```python
from build123d import *

# Parameters (mm, degrees)
BOSS_EXTRUDE1_DEPTH = 10
SKETCH4_R           = 7.5
CUT_EXTRUDE1_DEPTH  = 11
CHAMFER1_SIZE       = 1


with BuildPart() as part:
    # Sketch3 → Boss-Extrude1 (new body)
    with BuildSketch(Plane(origin=(0, 0, 0), x_dir=(1, 0, 0), z_dir=(0, 1, 0))):
        Polygon((-11, 6.350852961), (-11, -6.350852961), (0, -12.701705922), (11, -6.350852961), (11, 6.350852961), (0, 12.701705922), align=None)
    extrude(amount=BOSS_EXTRUDE1_DEPTH)

    # Sketch4 → Cut-Extrude1 (cut, through all)
    with BuildSketch(Plane(origin=(0, 10, 0), x_dir=(1, 0, 0), z_dir=(0, 1, 0))):
        Circle(SKETCH4_R)
    extrude(amount=-CUT_EXTRUDE1_DEPTH, mode=Mode.SUBTRACT)

    # Chamfer1
    chamfer1_edges = [part.edges().sort_by_distance(p)[0] for p in [
        (-7.5, 0, 0),
        (-7.5, 10, 0),
    ]]
    chamfer(chamfer1_edges, length=CHAMFER1_SIZE)

    # Sketch5 → Cut-Revolve1 (revolve, cut)
    with BuildSketch(Plane(origin=(0, 0, 0), x_dir=(0, 0, -1), z_dir=(1, 0, 0))):
        Polygon((-12.701705922, 10), (-12.701705922, 8.8), (-11.201705922, 10), align=None)
        Polygon((-12.701705922, 0), (-12.701705922, 1.2), (-11.201705922, 0), align=None)
    revolve(axis=Axis((0, 13.174691504, 0), (0, -1, 0)), mode=Mode.SUBTRACT)


solid = part.part
```
Geometry check sheet. Reference: the model listing, model coordinates, mm. Coordinates: 2 decimals unless noted, no trailing zeros. Loops run counter-clockwise (first coordinate to the right, second up) from the corner with the lowest first, then second, coordinate; pieces in that order, holes last. Notation, with made-up numbers: (13, 21.25) - (28, 21.25) arc R27 cw to (28, 37.25) - close; hole circle Ø10 at (-38.75, -18.5). An arc over 180 degrees is marked (long way). One line per item, written item: value. Start each with the question number.
(1) Depth check by flat-ended pin: P1, Ø5, axis at x = -4, z = 3.5, coming from the -Y side; P2, Ø1, axis at x = -5, z = 5.5, coming from the -Y side. Enter the tip coordinate at first touch or a pass-through.
(2) Cross-section at B-B on y = 2.5. Enter the section's corners in (x, z).
(3) Cross-section at A-A on z = 0. Enter the section's corners in (x, y).
(4) Material ranges on line 1 (X direction, y = 3.5, z = 0); line 2 (Z direction, x = 3.5, y = 2.75); line 3 (Z direction, x = -6.25, y = 6.5), recorded low to high. Write a range as [from, to].
Results below:
1. P1: stops at y = 0.68
1. P2: stops at y = 0.57
2. outline: (-11, -6.35) - (0, -12.7) - (11, -6.35) - (11, 6.35) - (0, 12.7) - (-11, 6.35) - close; hole circle Ø15 at (0, 0)
3. outline: (-11, 0) - (-8.5, 0) - (-7.5, 1) - (-7.5, 9) - (-8.5, 10) - (-11, 10) - close; (7.5, 1) - (8.5, 0) - (11, 0) - (11, 10) - (8.5, 10) - (7.5, 9) - close
4. line 1: x = [-11, -7.5], [7.5, 11]
4. line 2: z = [-10.68, -6.63], [6.63, 10.68]
4. line 3: z = [-9.09, -4.15], [4.15, 9.09]
